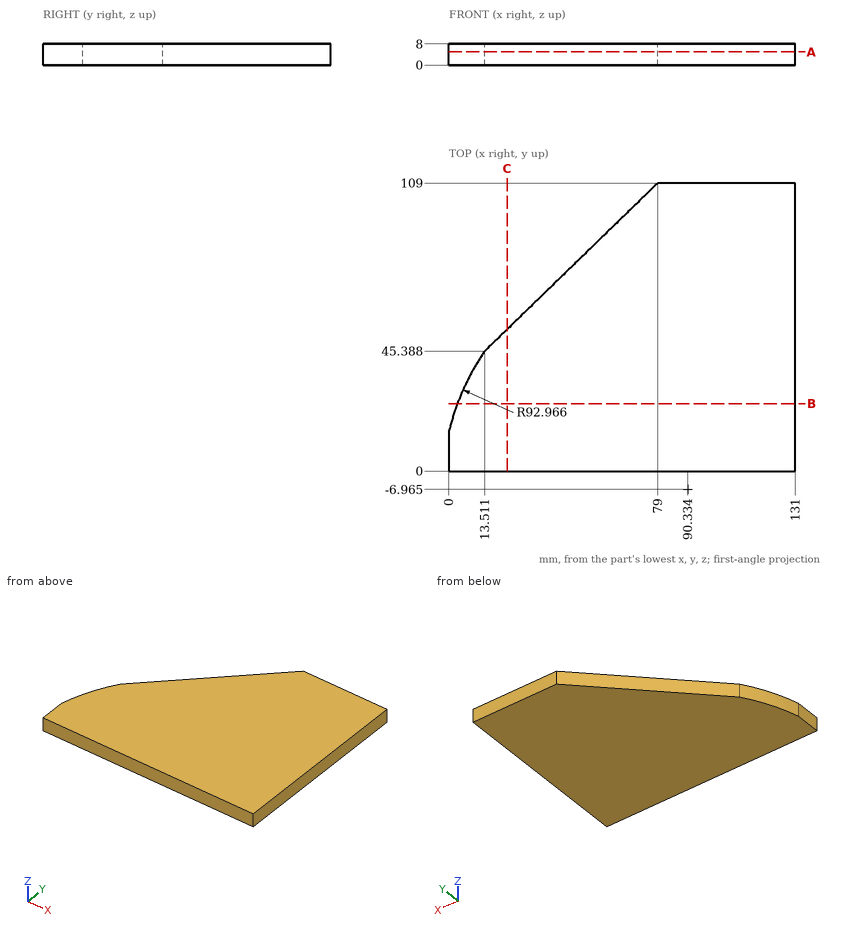
Can you work these out from the drawing? Everything is in mm from the part's minimum corner. Give positions to 0.01 mm unless a question says otherwise; leave off trailing zeros. Loops run counter-clockwise (first coordinate to the right, second up) from the corner with the lowest first, then second, coordinate; pieces in that order, holes last. Notation, with made-up numbers: M -11,5.25 L 4,5.25 A26 ccw 4,28.25 Z; hole C 42.25,55 d7. An arc over 180 degrees is marked long. Put each result on its own line as item: value. Start each with the question number.
(1) Will this pin go through, and if not, where does the flat tip stop? pin 1 Ø1.5 at (x, z) = (18, 3.5) entering from +Y.
(2) I need wall thicknesses on line 1 along X through (y, z) = (43, 4) (1 decimal); line 2 along Y through (x, z) = (60, 5.5) (1 decimal); line 3 along X through (y, z) = (15.5, 3.25). Which ranges of each line are inside material? Lowest first, please. Write a range as [from, to].
(3) I want a section at C-C on x = 22. Please give me the cut outline in (y, z) (1 decimal).
(4) I want a section at A-A on z = 5. Please give me the cut outline in (x, y) (1 decimal), then the cut area to 3 significant figures.
(5) I want a section at B-B on y = 25.5. Please give me the cut outline in (x, z), then the cut area to 3 significant figures.
Answer block:
1. pin 1: y = 50.48
2. line 1: [11.9, 131]
2. line 2: [0, 90.5]
2. line 3: [0.12, 131]
3. outline: M 0,0 L 53.6,0 L 53.6,8 L 0,8 Z
4. outline: M 0,0 L 131,0 L 131,109 L 79,109 L 13.5,45.4 A93 ccw 0,15 Z
4. area: 11,200 mm^2
5. outline: M 3.22,0 L 131,0 L 131,8 L 3.22,8 Z
5. area: 1,020 mm^2
